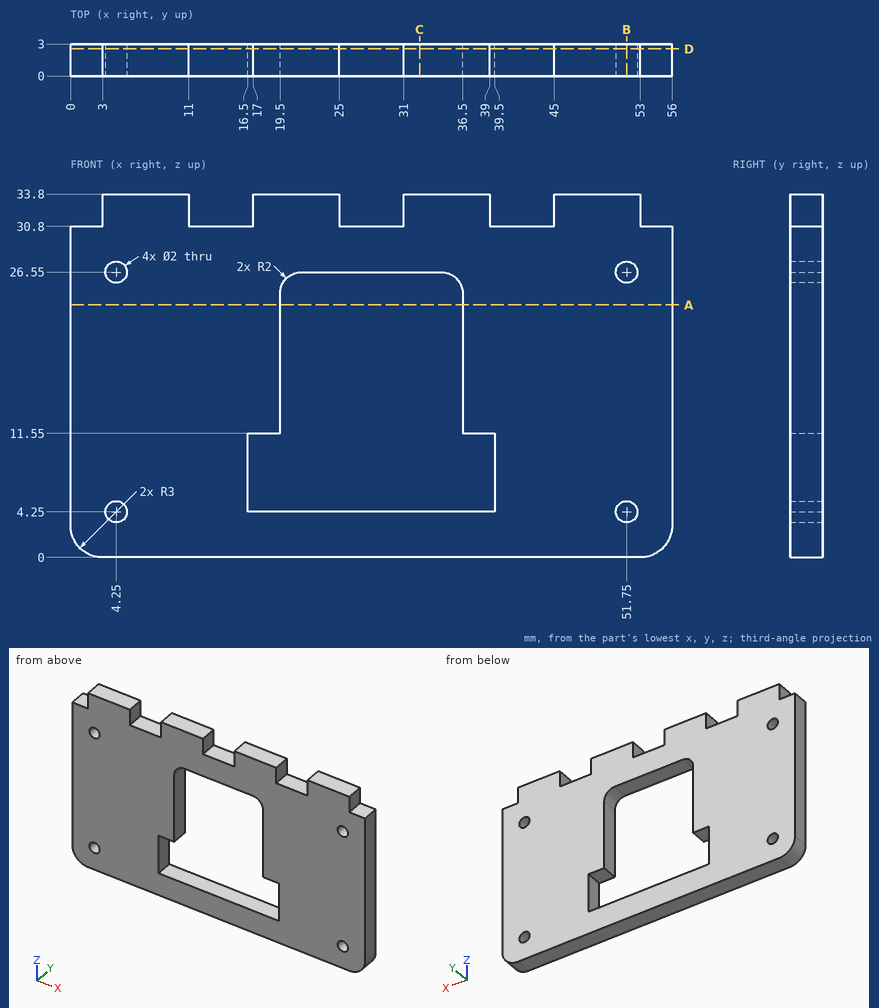
The figure shows three views and two pictorial views of one solid part (mm, origin at its lowest corner). Answer the questions. Round coordinates to 2 decimals unless told otherwise and drop trailing zeros. Order: outer loops, then holes, each group sorted by start corner. A loop starts at its lowest first (then second) coordinate and runs counter-clockwise, first axis right, second up. Notation, with made-up numbers: (-5, 57) - (22, 57) arc R15 cw to (22, 67) - close; hole circle Ø9 at (7.25, 83). An arc over 180 degrees is marked (long way). Write item = value, one per line. Start each with the question number.
1) Section B-B, the plane x = 51.75 is taken. Write down the section's boundary in (y, z).
2) Straight lines are drawn through the part: L1, parallel to Z at x = 51.75, y = 1; L2, parallel to X at y = 2.15, z = 32; L3, parallel to Z at x = 26, y = 1. For each, find the intervals that lie inside material, in ascending order.
3) Section D-D, the plane y = 2.55 is taken. Count the separate pieces of the cut face and the enclosed holes in it, plus the area to 3 significant figures.
4) Given pin 1 (1.5 mm diameter, centred on x = 27, y = 1.5, fed in from +Z), flat-ended and moving along its own axis, determine where the tip first touches the part or whether it passes through.
5) Section A-A, the plane z = 23.5 is taken. Write down the section's boundary in (x, y).
6) Section C-C, the plane x = 32.5 is taken. Write down the section's boundary in (y, z), plus the area to 3 significant figures.
Results list:
q1.outline = (0, 0) - (3, 0) - (3, 3.25) - (0, 3.25) - close; (0, 5.25) - (3, 5.25) - (3, 25.55) - (0, 25.55) - close; (0, 27.55) - (3, 27.55) - (3, 33.8) - (0, 33.8) - close
q2.L1 = 0 to 3.25, 5.25 to 25.55, 27.55 to 33.8
q2.L2 = 3 to 11, 17 to 25, 31 to 39, 45 to 53
q2.L3 = 0 to 4.25, 26.55 to 30.8
q3.separate_pieces = 1
q3.enclosed_holes = 5
q3.area = 1,380 mm^2
q4.pin_1 = 30.8
q5.outline = (0, 0) - (19.5, 0) - (19.5, 3) - (0, 3) - close; (36.5, 0) - (56, 0) - (56, 3) - (36.5, 3) - close
q6.outline = (0, 0) - (3, 0) - (3, 4.25) - (0, 4.25) - close; (0, 26.55) - (3, 26.55) - (3, 33.8) - (0, 33.8) - close
q6.area = 34.5 mm^2
